from build123d import *

# Parameters (mm, degrees)
SKETCH_1_R          = 4.5
EXTRUDE_1_DEPTH     = 10
CUT_EXTRUDE_1_REACH = 7
SKETCH_2_R          = 2
FILLET_2_R          = 1


with BuildPart() as part:
    # 草圖1 → 填料-伸長1 (new body)
    with BuildSketch(Plane.XY):
        with BuildLine():
            Line((7, -10), (7, 0))
            ThreePointArc((7, 0), (0, 7), (-7, 0))
            Line((-7, 0), (-7, -10))
            Line((-7, -10), (-17, -10))
            Line((-17, -10), (-17, -15))
            Line((-17, -15), (17, -15))
            Line((17, -15), (17, -10))
            Line((17, -10), (7, -10))
        make_face()
        Circle(SKETCH_1_R, mode=Mode.SUBTRACT)
    extrude(amount=EXTRUDE_1_DEPTH)

    # 草圖2 → 除料-伸長1 (cut, up to next)
    with BuildSketch(Plane(origin=(0, -10, 0), x_dir=(1, 0, 0), z_dir=(0, 1, 0)), mode=Mode.PRIVATE) as cut_extrude_1_sk1:
        with Locations((12, -5)):
            Circle(SKETCH_2_R)
    cut_extrude_1_tool1 = extrude(cut_extrude_1_sk1.sketch, amount=-CUT_EXTRUDE_1_REACH, mode=Mode.PRIVATE) & part.part
    add(cut_extrude_1_tool1.solids().sort_by_distance((12, -10, 5))[0], mode=Mode.SUBTRACT)
    # 草圖2 → 除料-伸長1 (cut, up to next)
    with BuildSketch(Plane(origin=(0, -10, 0), x_dir=(1, 0, 0), z_dir=(0, 1, 0)), mode=Mode.PRIVATE) as cut_extrude_1_sk2:
        with Locations((-12, -5)):
            Circle(SKETCH_2_R)
    cut_extrude_1_tool2 = extrude(cut_extrude_1_sk2.sketch, amount=-CUT_EXTRUDE_1_REACH, mode=Mode.PRIVATE) & part.part
    add(cut_extrude_1_tool2.solids().sort_by_distance((-12, -10, 5))[0], mode=Mode.SUBTRACT)

    # 圓角2
    fillet_2_edges = [part.edges().sort_by_distance(p)[0] for p in [
        (-17, -10, 5),
        (-7, -10, 5),
        (7, -10, 5),
        (17, -10, 5),
    ]]
    fillet(fillet_2_edges, radius=FILLET_2_R)


solid = part.part
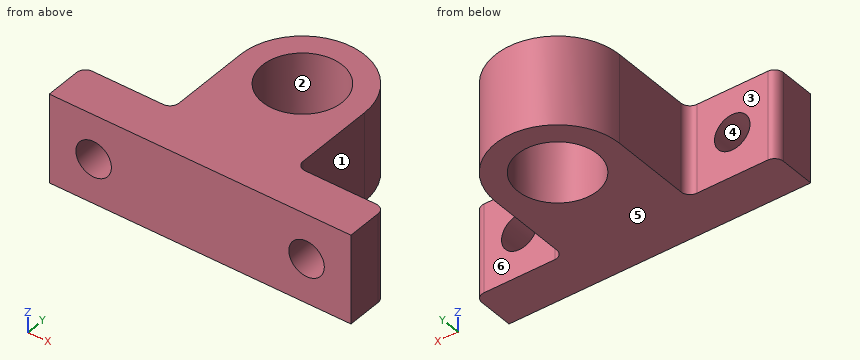
Work out the finished part from the listing and answer in its coordinate system (mm). Face numbers are marked on the shaded views. A direction names the side the tool comes from. Round coordinates to 2 decimals unless told otherwise and drop trailing zeros. Loops run counter-clockwise (first coordinate to the right, second up) from the corner with the lowest first, then second, coordinate; pieces in that order, holes last. Notation, with made-up numbers: M 70,25.5 L 87,25.5 A23 ccw 87,53.5 Z; hole C -14,47.25 d4. An arc over 180 degrees is marked long. One line per question, with ' | ' between items. Start each with the question number.
(1) For a pull along Z with two mould halves and no side action, classify the marked faces 4, 5 and 6 as released by +Z, released by -Z, zero draft, split by the parting line, or undercut.
(2) A cutting plane is placed at B-B on z = 5. Write down the section's boundary in (x, y), plus the area to 3 significant figures.
(3) Find the intervals of material crossed by line 1 (X direction, y = -12.15, z = 5); line 2 (Z direction, x = -12, y = -12.5); line 3 (Y direction, x = 0, z = 1.75), in increasing order.
(4) A cutting plane is placed at A-A on x = 0. Write down the section's boundary in (y, z).
(5) A cutting plane is placed at D-D on y = -3.5. Write down the section's boundary in (x, z).
(6) A cutting plane is placed at C-C on y = -12.5. Write down the section's boundary in (x, z).
(7) Flat-ended cylindrical pins translate along their axes: pin 1 Ø1.5 at (y, z) = (4.5, 1) entering from -X; pin 2 Ø1 at (x, z) = (3, 6) entering from +Y; pin 3 Ø10 at (x, y) = (12.5, -7) entering from +Z; pin 4 Ø5 at (y, z) = (-5, 3) entering from -X. Find the tip coordinate at first contact, or state that the pin passes through.
(8) A tool of negligible diameter and unlimited length cuts with its end or side. For the marked faces 1, 2 and 3, from which of +Z, -Z, +X, -X, +Y, -Y can it reach the whole face along a straight path? Write none if from no direction.
Geometry check:
1) face 4: undercut | face 5: released by -Z | face 6: zero draft
2) outline: M -17,-15 L -14,-15 L -14,-10 L -16,-10 A1 ccw -17,-11 Z; M -10,-15 L 10,-15 L 10,-10 L 8,-10 A1 cw 7,-9 L 7,0 A7 ccw -7,0 L -7,-9 A1 cw -8,-10 L -10,-10 Z; M 14,-15 L 17,-15 L 17,-11 A1 ccw 16,-10 L 14,-10 Z; hole C 0,0 d9 | area: 283 mm²
3) line 1: x = -17 to -14, -10 to 10, 14 to 17 | line 2: z = 0 to 3, 7 to 10 | line 3: y = -15 to -4.5, 4.5 to 7
4) outline: M -15,0 L -4.5,0 L -4.5,10 L -15,10 Z; M 4.5,0 L 7,0 L 7,10 L 4.5,10 Z
5) outline: M -7,0 L -2.83,0 L -2.83,10 L -7,10 Z; M 2.83,0 L 7,0 L 7,10 L 2.83,10 Z
6) outline: M -17,0 L 17,0 L 17,10 L -17,10 Z; hole C -12,5 d4; hole C 12,5 d4
7) pin 1: stops at x = -5.91 | pin 2: stops at y = 6.54 | pin 3: stops at z = 10 | pin 4: stops at x = -7
8) face 1: +Z, -Z, +X, +Y | face 2: +Z, -Z | face 3: +Z, -Z, -X, +Y
